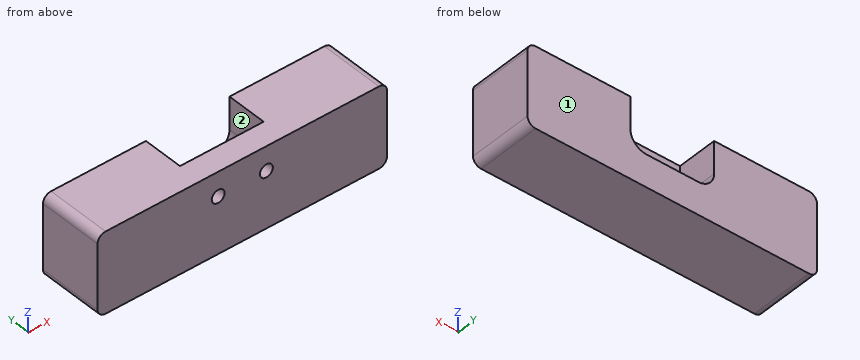
```python
from build123d import *

# Parameters (mm, degrees)
ESBO_O2_W                                  = 36
ESBO_O2_H                                  = 10
RESSALTO_EXTRUS_O2_DEPTH                   = 8
FILETE3_R                                  = 1
ESBO_O5_W                                  = 10.4
ESBO_O5_H                                  = 6
CORTE_EXTRUS_O1_DEPTH                      = 5
FILETE4_R                                  = 2
BROCA_DE_ROSQUEAR_PARA_TARRAXA_DE_M2X0_4_D = 1.6


with BuildPart() as part:
    # Esboço2 → Ressalto-extrusão2 (new body)
    with BuildSketch(Plane(origin=(0, 0, 0), x_dir=(1, 0, 0), z_dir=(0, 1, 0))):
        with Locations((15, 5)):
            Rectangle(ESBO_O2_W, ESBO_O2_H)
    extrude(amount=RESSALTO_EXTRUS_O2_DEPTH)

    # Filete3
    filete3_edges = [part.edges().sort_by_distance(p)[0] for p in [
        (33, 4, 0),
        (-3, 4, 0),
        (-3, 4, -10),
        (33, 4, -10),
    ]]
    fillet(filete3_edges, radius=FILETE3_R)

    # Esboço5 → Corte-extrusão1 (cut)
    with BuildSketch(Plane(origin=(0, 8, 0), x_dir=(1, 0, 0), z_dir=(0, 1, 0))):
        with Locations((15, 3)):
            Rectangle(ESBO_O5_W, ESBO_O5_H)
    extrude(amount=-CORTE_EXTRUS_O1_DEPTH, mode=Mode.SUBTRACT)

    # Filete4
    filete4_edges = [part.edges().sort_by_distance(p)[0] for p in [
        (20.2, 5.5, -6),
        (9.8, 5.5, -6),
    ]]
    fillet(filete4_edges, radius=FILETE4_R)

    # Broca de rosquear para tarraxa de M2x0.41 (through all)
    with Locations(Plane(origin=(12, 3, -3), x_dir=(0, 0, 1), z_dir=(0, 1, 0))):
        with Locations((0, 0), (0, 6)):
            Hole(BROCA_DE_ROSQUEAR_PARA_TARRAXA_DE_M2X0_4_D / 2)


solid = part.part
```
The model under review builds one solid part; all positions refer to its coordinate system, in mm. Face numbers are marked on the shaded views. A direction names the side the tool comes from. Round coordinates to 2 decimals unless told otherwise and drop trailing zeros. Write each loop counter-clockwise with the first axis right and the second up, starting at its lowest first coordinate (ties: lowest second). Pieces come first, ordered by that corner, then holes.
(1) We need section A-A on z = -3. Give the boundary of the cut face in (x, y), and give its area (3 significant figures).
(2) Insertion check: pin 1 (3 mm diameter, centred on x = 15.5, z = -3, fed in from +Y); pin 2 (1.5 mm diameter, centred on x = 14.5, y = 4.5, fed in from +Z). Each pin has a flat end and moves straight along its axis. Give the tip position at first contact, or say it passes through.
(3) We need section C-C on x = 13.5. Give the boundary of the cut face in (y, z).
(4) We need section D-D on z = -5. Give the boundary of the cut face in (x, y).
(5) We need section B-B on y = 6. Give the boundary of the cut face in (x, z).
(6) Wall thickness on L1, parallel to X at y = 1.4, z = -3; L2, parallel to X at y = 5.75, z = -4; L3, parallel to Y at x = 20, z = -4.75: over which ranges is each line inside the solid? List them lowest first.
(7) Machinability: for the marked faces 1 and 2, which of the approach directions +Z, -Z, +X, -X, +Y, -Y give a long, thin tool a straight path to every point of the face, cutting with its end or side? Answer none if there is none.
Findings below:
1. outline: (-3, 0) - (11.2, 0) - (11.2, 3) - (9.8, 3) - (9.8, 8) - (-3, 8) - close; (12.8, 0) - (17.2, 0) - (17.2, 3) - (12.8, 3) - close; (18.8, 0) - (33, 0) - (33, 8) - (20.2, 8) - (20.2, 3) - (18.8, 3) - close
1. area: 226 mm2
2. pin 1: stops at y = 3
2. pin 2: stops at z = -6
3. outline: (0, -10) - (8, -10) - (8, -6) - (3, -6) - (3, 0) - (0, 0) - close
4. outline: (-3, 0) - (33, 0) - (33, 8) - (19.93, 8) - (19.93, 3) - (10.07, 3) - (10.07, 8) - (-3, 8) - close
5. outline: (-3, -9) arc R1 ccw to (-2, -10) - (32, -10) arc R1 ccw to (33, -9) - (33, -1) arc R1 ccw to (32, 0) - (20.2, 0) - (20.2, -4) arc R2 cw to (18.2, -6) - (11.8, -6) arc R2 cw to (9.8, -4) - (9.8, 0) - (-2, 0) arc R1 ccw to (-3, -1) - close
6. L1: x = -3 to 11.2, 12.8 to 17.2, 18.8 to 33
6. L2: x = -3 to 9.8, 20.2 to 33
6. L3: y = 0 to 3
7. face 1: +Z, -Z, +X, -X, +Y
7. face 2: +Z, +Y
